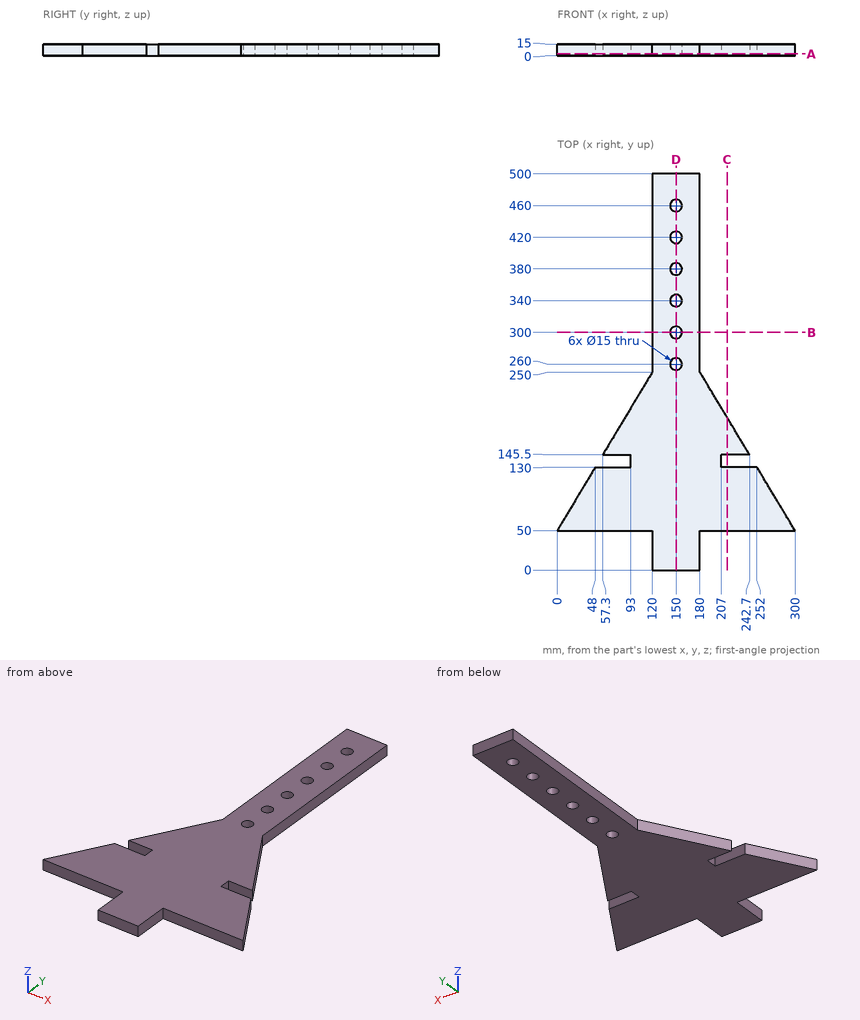
Job drawing, mm, ordinate dimensions from the low corner. One solid piece. Give positions to 0.01 mm unless a question says otherwise; leave off trailing zeros. Loops run counter-clockwise (first coordinate to the right, second up) from the corner with the lowest first, then second, coordinate; pieces in that order, holes last. Notation, with made-up numbers: (-15.5, 41) -> (26.5, 41) arc R20 cw to (26.5, 55) -> close; hole circle Ø1 at (61.25, 58.5). An arc over 180 degrees is marked (long way). Use a Markdown table: item, result. Add a question column.
(1) Slice it at D-D on x = 150. List the corners of the cut face in (y, z).
(2) Slice it at A-A on z = 2.5. List the corners of the cut face in (x, y).
(3) Wall check: line 1 along X through (y, z) = (300, 5.5); line 2 along X through (y, z) = (368, 9.75); line 3 along X through (y, z) = (306, 9). Give the ranges that are in metal, low to high.
(4) Slice it at B-B on y = 300. List the corners of the cut face in (x, z).
(5) Drop flat-ended pins along their axis: pin 1 Ø1 at (y, z) = (349.5, 4) entering from +X; pin 2 Ø10 at (x, y) = (267, 119) entering from +Z; pin 3 Ø7.5 at (x, z) = (223, 6) entering from -Y; pin 4 Ø3 at (y, z) = (441, 2) entering from -X. Give the stop position or say it passes through.
(6) Slice it at C-C on x = 214.5. List the corners of the cut face in (y, z), and give its area (4 significant figures).
Filled sheet:
| question | item | result |
|---|---|---|
| 1 | outline | (0, 0) -> (252.5, 0) -> (252.5, 15) -> (0, 15) -> close; (267.5, 0) -> (292.5, 0) -> (292.5, 15) -> (267.5, 15) -> close; (307.5, 0) -> (332.5, 0) -> (332.5, 15) -> (307.5, 15) -> close; (347.5, 0) -> (372.5, 0) -> (372.5, 15) -> (347.5, 15) -> close; (387.5, 0) -> (412.5, 0) -> (412.5, 15) -> (387.5, 15) -> close; (427.5, 0) -> (452.5, 0) -> (452.5, 15) -> (427.5, 15) -> close; (467.5, 0) -> (500, 0) -> (500, 15) -> (467.5, 15) -> close |
| 2 | outline | (0, 50) -> (120, 50) -> (120, 0) -> (180, 0) -> (180, 50) -> (300, 50) -> (252, 130) -> (207, 130) -> (207, 145.5) -> (242.7, 145.5) -> (180, 250) -> (180, 500) -> (120, 500) -> (120, 250) -> (57.3, 145.5) -> (93, 145.5) -> (93, 130) -> (48, 130) -> close; hole circle Ø15 at (150, 260); hole circle Ø15 at (150, 300); hole circle Ø15 at (150, 340); hole circle Ø15 at (150, 380); hole circle Ø15 at (150, 420); hole circle Ø15 at (150, 460) |
| 3 | line 1 | 120 to 142.5, 157.5 to 180 |
| 3 | line 2 | 120 to 180 |
| 3 | line 3 | 120 to 145.5, 154.5 to 180 |
| 4 | outline | (120, 0) -> (142.5, 0) -> (142.5, 15) -> (120, 15) -> close; (157.5, 0) -> (180, 0) -> (180, 15) -> (157.5, 15) -> close |
| 5 | pin 1 | x = 180 |
| 5 | pin 2 | through |
| 5 | pin 3 | y = 50 |
| 5 | pin 4 | x = 120 |
| 6 | outline | (50, 0) -> (130, 0) -> (130, 15) -> (50, 15) -> close; (145.5, 0) -> (192.5, 0) -> (192.5, 15) -> (145.5, 15) -> close |
| 6 | area | 1,905 mm2 |
